Model file for the job. Use its own axes, mm. A direction names the side the tool comes from. Round coordinates to 2 decimals unless told otherwise and drop trailing zeros. Loops run counter-clockwise (first coordinate to the right, second up) from the corner with the lowest first, then second, coordinate; pieces in that order, holes last. Notation, with made-up numbers: (-23, 84) -> (-8, 84) arc R11 cw to (-8, 89) -> close; hole circle Ø11 at (-15.5, 23). An arc over 180 degrees is marked (long way). Use a Markdown table: item, result.
from build123d import *

# Parameters (mm, degrees)
SKETCH_2_W          = 10
SKETCH_2_H          = 5
EXTRUDE_1_DEPTH     = 1.5
SKETCH_3_R          = 1.55
CUT_EXTRUDE_1_DEPTH = 1.5
SKETCH_4_W          = 5
SKETCH_4_H          = 5
EXTRUDE_2_DEPTH     = 125
SKETCH_5_W          = 10
SKETCH_5_H          = 5
EXTRUDE_3_DEPTH     = 1.5
SKETCH_6_R          = 1.55
CUT_EXTRUDE_2_DEPTH = 1.5
SKETCH_7_R          = 1.5
EXTRUDE_4_DEPTH     = 2
EXTRUDE_START       = 2
SKETCH_8_R          = 1.5
EXTRUDE_5_DEPTH     = 2


with BuildPart() as part:
    # 草图2 → 凸台-拉伸1 (new body)
    with BuildSketch(Plane(origin=(0, 0, 0), x_dir=(1, 0, 0), z_dir=(0, 1, 0))):
        Rectangle(SKETCH_2_W, SKETCH_2_H)
    extrude(amount=EXTRUDE_1_DEPTH)

    # 草图3 → 切除-拉伸1 (cut)
    with BuildSketch(Plane.XZ):
        with Locations(Location((-2.5, 0, 0), (0, 0, 270))):
            Circle(SKETCH_3_R)
    extrude(amount=-CUT_EXTRUDE_1_DEPTH, mode=Mode.SUBTRACT)

    # 草图4 → 凸台-拉伸2 (add)
    with BuildSketch(Plane.XZ):
        with Locations((2.5, 0)):
            Rectangle(SKETCH_4_W, SKETCH_4_H)
    extrude(amount=EXTRUDE_2_DEPTH)

    # 草图5 → 凸台-拉伸3 (add)
    with BuildSketch(Plane.XZ.offset(125)):
        Rectangle(SKETCH_5_W, SKETCH_5_H)
    extrude(amount=EXTRUDE_3_DEPTH)

    # 草图6 → 切除-拉伸2 (cut)
    with BuildSketch(Plane.XZ.offset(126.5)):
        with Locations(Location((-2.5, 0, 0), (0, 0, 270))):
            Circle(SKETCH_6_R)
    extrude(amount=-CUT_EXTRUDE_2_DEPTH, mode=Mode.SUBTRACT)

    # 草图7 → 凸台-拉伸4 (add)
    with BuildSketch(Plane(origin=(0, 1.5, 0), x_dir=(1, 0, 0), z_dir=(0, 1, 0))):
        with Locations(Location((2.5, 0, 0), (0, 0, 270))):
            Circle(SKETCH_7_R)
    extrude(amount=EXTRUDE_4_DEPTH)

    # 草图8 → 凸台-拉伸5 (add)
    with BuildSketch(Plane.XZ.offset(126.5).offset(EXTRUDE_START)):
        with Locations(Location((2.5, 0, 0), (0, 0, 90))):
            Circle(SKETCH_8_R)
    extrude(amount=-EXTRUDE_5_DEPTH)


solid = part.part
Q1. Pull direction X, two halves, no side cores. Call faces 1 (the face through (-3.875, -125.76, -0.715)), 2 (the face through (-3.875, 0.74, -0.715)), 3 (the face through (5, -62, 0)), 4 (the face through (0, 1.5, 0)): released by +X, released by -X, zero draft, split by the parting line, or undercut.
Results list:
| item | result |
|---|---|
| face 1 | undercut |
| face 2 | undercut |
| face 3 | released by +X |
| face 4 | zero draft |
Q2. Band-saw the part on A-A, the plane x = -2.5. Give the cut face in (y, z).
Results list:
| item | result |
|---|---|
| outline | (-126.5, -2.5) -> (-125, -2.5) -> (-125, -1.55) -> (-126.5, -1.55) -> close; (-126.5, 1.55) -> (-125, 1.55) -> (-125, 2.5) -> (-126.5, 2.5) -> close; (0, -2.5) -> (1.5, -2.5) -> (1.5, -1.55) -> (0, -1.55) -> close; (0, 1.55) -> (1.5, 1.55) -> (1.5, 2.5) -> (0, 2.5) -> close |
Q3. Drill centre lines: L1, parallel to X at y = -126, z = 0; L2, parallel to Y at x = -2, z = -2.2; L3, parallel to X at y = -15.5, z = -1.35. Where is each one in solid material? Low to high. Write a range as from..to.
Results list:
| item | result |
|---|---|
| L1 | x = -5..-4.05, -0.95..5 |
| L2 | y = -126.5..-125, 0..1.5 |
| L3 | x = 0..5 |
Q4. Band-saw the part on B-B, the plane z = 0. Give the cut face in (x, y), plus the area to 3 significant figures.
Results list:
| item | result |
|---|---|
| outline | (-5, -126.5) -> (-4.05, -126.5) -> (-4.05, -125) -> (-5, -125) -> close; (-5, 0) -> (-4.05, 0) -> (-4.05, 1.5) -> (-5, 1.5) -> close; (-0.95, -126.5) -> (1, -126.5) -> (1, -128.5) -> (4, -128.5) -> (4, -126.5) -> (5, -126.5) -> (5, 1.5) -> (4, 1.5) -> (4, 3.5) -> (1, 3.5) -> (1, 1.5) -> (-0.95, 1.5) -> (-0.95, 0) -> (0, 0) -> (0, -125) -> (-0.95, -125) -> close |
| area | 658 mm² |
Q5. Band-saw the part on C-C, the plane y = -106. Give the cut face in (x, z).
Results list:
| item | result |
|---|---|
| outline | (0, -2.5) -> (5, -2.5) -> (5, 2.5) -> (0, 2.5) -> close |
Q6. Flat gauge pins, fed straight in: pin 1 (2.5 mm diameter, centred on x = -1.5, z = 0, fed in from +Y); pin 2 (1.5 mm diameter, centred on x = -1, z = 0.5, fed in from -Y). Where does each tip first touch, or does it go through?
Results list:
| item | result |
|---|---|
| pin 1 | stops at y = 1.5 |
| pin 2 | stops at y = -126.5 |
Q7. Tool access for faces 5 (the face through (1, 2, 0)), 6 (the face through (0, -62, 0)), 7 (the face through (3.83, -127.51, 0.69)): list every direction of +Z, -Z, +X, -X, +Y, -Y with a clear straight run to the whole face (end or side of a thin tool).
Results list:
| item | result |
|---|---|
| face 5 | +Y |
| face 6 | +Z, -Z, -X |
| face 7 | -Y |
